Geometry check sheet. Reference: the model listing, model coordinates, mm. A direction names the side the tool comes from. Round coordinates to 2 decimals unless told otherwise and drop trailing zeros. Order: outer loops, then holes, each group sorted by start corner. A loop starts at its lowest first (then second) coordinate and runs counter-clockwise, first axis right, second up. Notation, with made-up numbers: (22, 17) -> (68, 17) arc R11 cw to (68, 24) -> close; hole circle Ø3 at (38, 3.25). An arc over 180 degrees is marked (long way). Use a Markdown table: item, result. Add a question column.
Item 1: Material ranges on probe 1 along Y at (x, z) = (32, 2); probe 2 along X at (y, z) = (41, -2.75); probe 3 along X at (y, z) = (34, 1.75), recorded low to high. Write a range as [from, to].
Item 2: Sectioned sample at D-D, the plane z = 2.25. State how many separate pieces and enclosed holes the cut face has, and give its area (3 significant figures).
Item 3: Gauge pin test, flat ends, axial feed: pin 1 Ø3.5 at (x, y) = (46.85, 41.23) entering from -Z; pin 2 Ø1 at (x, y) = (18.5, 15.5) entering from -Z. Record the tip position at first contact, or that the pin passes through.
Item 4: Mould release check, pull along X, two halves, no side actions. Record for faces 1 (the cylindrical face through (45.4, -24.21, -3.41)), 2 (the flat face through (28, -29.274, -8)), 3 (the flat face through (51.85, 9, -3)): pulls with the +X half, pulls with the -X half, needs draft (parallel to the pull), parting line crosses it, or undercut.
Item 5: Sectioned sample at C-C, the plane z = -9. Record the cut outline in (x, y).
Item 6: Sectioned sample at A-A, the plane y = -12. Record the cut outline in (x, z).
Item 7: Set-up check for faces 4 (the flat face through (40, -24, -4)), 5 (the flat face through (41.85, 9, -5)), 6 (the flat face through (27, -2.748, 1)): record each of +Z, -Z, +X, -X, +Y, -Y from which the full face is reachable in a straight line by a thin tool's end or side.
Item 8: Sectioned sample at B-B, the plane z = -5.25. Record the cut outline in (x, y), and give its area (3 significant figures).
Autodesk Fusion 360 part; units mm, degrees
sketch "Sketch1" plane through (0, 0, 0) normal (0, 0, 1) x (1, 0, 0)
  line L0 (12.8502, 36.2265) -> (41.8502, 36.2265)
  line L1 (41.8502, 36.2265) -> (41.8502, -19.2735)
  line L2 (41.8502, -19.2735) -> (12.8502, -19.2735)
  line L3 (12.8502, -19.2735) -> (12.8502, 36.2265)
  line L4 (51.8502, 46.2265) -> (51.8502, -29.2735)
  line L5 (51.8502, -29.2735) -> (2.8502, -29.2735)
  line L6 (2.8502, -29.2735) -> (2.8502, 46.2265)
  line L7 (2.8502, 46.2265) -> (51.8502, 46.2265)
  line L8 (51.8502, -29.2735) -> (46.8502, -29.2735)
  line L9 (46.8502, -29.2735) -> (46.8502, 46.2265)
  line L10 (51.8502, -29.2735) -> (51.8502, -24.2735)
  line L11 (51.8502, -24.2735) -> (2.8502, -24.2735)
  line L12 (2.8502, -29.2735) -> (7.8502, -29.2735)
  line L13 (7.8502, -29.2735) -> (7.8502, 46.2265)
  line L14 (2.8502, 46.2265) -> (2.8502, 41.2265)
  line L15 (2.8502, 41.2265) -> (51.8502, 41.2265)
  circle A0 centre (46.8502, -24.2735) radius 1.45
  circle A1 centre (7.8502, -24.2735) radius 1.45
  circle A2 centre (46.8502, 41.2265) radius 1.45
  circle A3 centre (7.8502, 41.2265) radius 1.45
  line L16 (41.8502, -19.2735) -> (27.3502, -19.2735)
  line L17 (36.8752, -19.2735) -> (36.8752, 37.8765)
  line L18 (34.3502, 2.8015) -> (34.3502, 15.8015)
  line L19 (20.3502, 2.8015) -> (20.3502, 15.8015)
  line L20 (17.8252, -19.2735) -> (17.8252, 37.8765)
  line L21 (17.8252, -19.2735) -> (17.8252, 37.8765)
  line L22 (34.3502, 2.8015) -> (34.3502, 15.8015)
  line L23 (20.3502, 2.8015) -> (20.3502, 15.8015)
  line L24 (34.3502, -16.2485) -> (34.3502, -3.2485)
  arc A4 (20.3502, 2.8015) -> (20.8502, 2.3015) centre (20.8502, 2.8015) ccw
  arc A5 (34.3502, 34.8515) -> (33.8502, 35.3515) centre (33.8502, 34.8515) ccw
  line L25 (36.8752, -19.2735) -> (36.8752, 37.8765)
  arc A6 (20.3502, -16.2485) -> (20.8502, -16.7485) centre (20.8502, -16.2485) ccw
  arc A7 (33.8502, -16.7485) -> (34.3502, -16.2485) centre (33.8502, -16.2485) ccw
  line L26 (20.8502, -2.7485) -> (33.8502, -2.7485)
  line L27 (36.8752, -19.2735) -> (17.8252, -19.2735)
  line L28 (20.8502, 21.3515) -> (33.8502, 21.3515)
  arc A8 (33.8502, -16.7485) -> (34.3502, -16.2485) centre (33.8502, -16.2485) ccw
  line L29 (34.3502, -16.2485) -> (34.3502, -3.2485)
  line L30 (20.8502, 35.3515) -> (33.8502, 35.3515)
  line L31 (36.8752, 37.8765) -> (17.8252, 37.8765)
  line L32 (20.8502, 35.3515) -> (33.8502, 35.3515)
  arc A9 (20.8502, -2.7485) -> (20.3502, -3.2485) centre (20.8502, -3.2485) ccw
  line L33 (20.8502, 2.3015) -> (33.8502, 2.3015)
  arc A10 (20.3502, 21.8515) -> (20.8502, 21.3515) centre (20.8502, 21.8515) ccw
  arc A11 (33.8502, 2.3015) -> (34.3502, 2.8015) centre (33.8502, 2.8015) ccw
  arc A12 (20.8502, -2.7485) -> (20.3502, -3.2485) centre (20.8502, -3.2485) ccw
  line L34 (20.3502, -16.2485) -> (20.3502, -3.2485)
  line L35 (20.8502, -2.7485) -> (33.8502, -2.7485)
  arc A13 (34.3502, -3.2485) -> (33.8502, -2.7485) centre (33.8502, -3.2485) ccw
  line L36 (20.3502, 21.8515) -> (20.3502, 34.8515)
  arc A14 (34.3502, 34.8515) -> (33.8502, 35.3515) centre (33.8502, 34.8515) ccw
  arc A15 (20.3502, 21.8515) -> (20.8502, 21.3515) centre (20.8502, 21.8515) ccw
  arc A16 (20.3502, -16.2485) -> (20.8502, -16.7485) centre (20.8502, -16.2485) ccw
  line L37 (36.8752, -19.2735) -> (17.8252, -19.2735)
  line L38 (36.8752, 37.8765) -> (17.8252, 37.8765)
  arc A17 (20.3502, 2.8015) -> (20.8502, 2.3015) centre (20.8502, 2.8015) ccw
  line L39 (20.3502, -16.2485) -> (20.3502, -3.2485)
  arc A18 (34.3502, -3.2485) -> (33.8502, -2.7485) centre (33.8502, -3.2485) ccw
  arc A19 (34.3502, 15.8015) -> (33.8502, 16.3015) centre (33.8502, 15.8015) ccw
  arc A20 (20.8502, 35.3515) -> (20.3502, 34.8515) centre (20.8502, 34.8515) ccw
  arc A21 (34.3502, 15.8015) -> (33.8502, 16.3015) centre (33.8502, 15.8015) ccw
  line L40 (34.3502, 21.8515) -> (34.3502, 34.8515)
  line L41 (20.8502, -16.7485) -> (33.8502, -16.7485)
  line L42 (20.8502, 21.3515) -> (33.8502, 21.3515)
  line L43 (20.3502, 21.8515) -> (20.3502, 34.8515)
  line L44 (20.8502, 2.3015) -> (33.8502, 2.3015)
  line L45 (34.3502, 21.8515) -> (34.3502, 34.8515)
  arc A22 (33.8502, 2.3015) -> (34.3502, 2.8015) centre (33.8502, 2.8015) ccw
  arc A23 (20.8502, 35.3515) -> (20.3502, 34.8515) centre (20.8502, 34.8515) ccw
  line L46 (20.8502, -16.7485) -> (33.8502, -16.7485)
  arc A24 (20.8502, 16.3015) -> (20.3502, 15.8015) centre (20.8502, 15.8015) ccw
  arc A25 (33.8502, 21.3515) -> (34.3502, 21.8515) centre (33.8502, 21.8515) ccw
  line L47 (20.8502, 16.3015) -> (33.8502, 16.3015)
  arc A26 (33.8502, 21.3515) -> (34.3502, 21.8515) centre (33.8502, 21.8515) ccw
  arc A27 (20.8502, 16.3015) -> (20.3502, 15.8015) centre (20.8502, 15.8015) ccw
  line L48 (20.8502, 16.3015) -> (33.8502, 16.3015)
  line L49 (36.8752, -19.2735) -> (28.3002, -19.2735)
  line L50 (36.8752, -19.2735) -> (27.3502, -19.2735)
  dimension "d1" = 29
  dimension "d2" = 55.5
  dimension "d3" = -10
  dimension "d4" = 5
  dimension "d5" = 5
  dimension "d6" = 5
  dimension "d7" = 5
  dimension "d8" = 2.9
  dimension "d9" = 2.9
  dimension "d10" = 2.9
  dimension "d11" = 2.9
extrude "Extrude1" add sketch "Sketch1" along normal blind 3 contours L0 L2 L3 L20 L21 | L0 L17 L20 L21 L25 L31 L38 | L0 L2 L16 L17 L20 L21 L25 L27 L37 L49 L50 | L0 L1 L2 L16 L17 L25 | L4 L7 L9 L15 A2 | L4 L9 L11 L15 A0 A2 | L7 L9 L13 L15 A2 A3 | L4 L5 L8 L9 L10 L11 A0 | L6 L7 L13 L14 L15 A3 | L9 L11 L13 L15 A0 A1 A2 A3 | L5 L9 L11 L13 A0 A1 | L6 L11 L13 L15 A1 A3 | L5 L6 L11 L12 L13 A1 | L18 L19 L22 L23 A4 L33 A11 A17 A19 A21 L44 A22 A24 L47 A27 L48 | L24 A6 A7 L26 A8 L29 A9 A12 L34 L35 A13 A16 L39 A18 L41 L46 | A5 L28 L30 L32 A10 L36 A14 A15 A20 L40 L42 L43 L45 A23 A25 A26
extrude "Extrude2" add sketch "Sketch1" against normal blind 10 contours L0 L17 L20 L21 L25 L31 L38 | L4 L7 L9 L15 A2 | L4 L9 L11 L15 A0 A2 | L7 L9 L13 L15 A2 A3 | L4 L5 L8 L9 L10 L11 A0 | L6 L7 L13 L14 L15 A3 | L9 L11 L13 L15 A0 A1 A2 A3 | L5 L9 L11 L13 A0 A1 | L6 L11 L13 L15 A1 A3 | L5 L6 L11 L12 L13 A1
extrude "Extrude3" cut sketch "Sketch1" along normal blind 10 contours L18 L19 L22 L23 A4 L33 A11 A17 A19 A21 L44 A22 A24 L47 A27 L48 | L24 A6 A7 L26 A8 L29 A9 A12 L34 L35 A13 A16 L39 A18 L41 L46 | A5 L28 L30 L32 A10 L36 A14 A15 A20 L40 L42 L43 L45 A23 A25 A26
sketch "Sketch3" plane through (0, -29.2735, 0) normal (0, -1, 0) x (1, 0, 0)
  line L0 (51.8502, -10) -> (51.8502, 3)
  line L1 (51.8502, 3) -> (2.8502, 3)
  line L2 (2.8502, 3) -> (2.8502, -10)
  line L3 (2.8502, -10) -> (51.8502, -10)
  line L4 (40, 0) -> (15, 0)
  line L5 (15, 0) -> (15, -7)
  line L6 (15, -7) -> (40, -7)
  line L7 (40, -7) -> (40, 0)
extrude "Extrude4" cut sketch "Sketch3" against normal blind 19 contours L4 L5 L6 L7
Found:
| question | item | result |
|---|---|---|
| 1 | probe 1 | y = [-29.27, -16.75], [-2.75, 2.3], [16.3, 21.35], [35.35, 46.23] |
| 1 | probe 2 | x = [2.85, 6.42], [9.28, 45.42], [48.28, 51.85] |
| 1 | probe 3 | x = [2.85, 20.35], [34.35, 51.85] |
| 2 | separate pieces | 1 |
| 2 | enclosed holes | 7 |
| 2 | area | 3,090 mm2 |
| 3 | pin 1 | stops at z = -10 |
| 3 | pin 2 | stops at z = 0 |
| 4 | face 1 | undercut |
| 4 | face 2 | needs draft |
| 4 | face 3 | pulls with the +X half |
| 5 | outline | (2.85, -29.27) -> (51.85, -29.27) -> (51.85, 46.23) -> (2.85, 46.23) -> close; hole circle Ø2.9 at (7.85, -24.27); hole circle Ø2.9 at (7.85, 41.23); hole (12.85, -19.27) -> (41.85, -19.27) -> (41.85, 36.23) -> (12.85, 36.23) -> close; hole circle Ø2.9 at (46.85, -24.27); hole circle Ø2.9 at (46.85, 41.23) |
| 6 | outline | (2.85, -10) -> (12.85, -10) -> (12.85, 0) -> (20.35, 0) -> (20.35, 3) -> (2.85, 3) -> close; (34.35, 0) -> (41.85, 0) -> (41.85, -10) -> (51.85, -10) -> (51.85, 3) -> (34.35, 3) -> close |
| 7 | face 4 | -Y |
| 7 | face 5 | -Z |
| 7 | face 6 | +Z, -Z |
| 8 | outline | (2.85, -29.27) -> (15, -29.27) -> (15, -19.27) -> (12.85, -19.27) -> (12.85, 36.23) -> (41.85, 36.23) -> (41.85, -19.27) -> (40, -19.27) -> (40, -29.27) -> (51.85, -29.27) -> (51.85, 46.23) -> (2.85, 46.23) -> close; hole circle Ø2.9 at (7.85, -24.27); hole circle Ø2.9 at (7.85, 41.23); hole circle Ø2.9 at (46.85, -24.27); hole circle Ø2.9 at (46.85, 41.23) |
| 8 | area | 1,810 mm2 |
